```python
from build123d import *

# Parameters (mm, degrees)
ESQUISSE2_W        = 10
ESQUISSE2_H        = 8
BOSS_EXTRU_1_START = -10
BOSS_EXTRU_1_DEPTH = 10


with BuildPart() as part:
    # Esquisse2 → Révolution1 (revolve)
    with BuildSketch(Plane(origin=(0, 0, 0), x_dir=(0, 0, -1), z_dir=(1, 0, 0)), mode=Mode.PRIVATE) as r_volution1_sk:
        with Locations((5, 7)):
            Rectangle(ESQUISSE2_W, ESQUISSE2_H)
    revolve(r_volution1_sk.sketch.rotate(Axis((0, 0, 0), (0, 0, -1)), 90), axis=Axis((0, 0, 0), (0, 0, -1)))

    # Esquisse3 → Boss.-Extru.1 (add)
    with BuildSketch(Plane.XY.offset(BOSS_EXTRU_1_START)):
        with BuildLine():
            Line((0, 14), (-1.5, 10.897247359))
            ThreePointArc((-1.5, 10.897247359), (-0.751757625, 10.974281775), (0, 11))
            ThreePointArc((0, 11), (0.751757625, 10.974281775), (1.5, 10.897247359))
            Line((1.5, 10.897247359), (0, 14))
        make_face()
        with BuildLine():
            Line((3.944255796, 13.432901631), (4.509348821, 10.033233437))
            ThreePointArc((4.509348821, 10.033233437), (3.813118623, 10.317951656), (3.099058125, 10.55442271))
            ThreePointArc((3.099058125, 10.55442271), (2.370506305, 10.741540851), (1.630869901, 10.878431108))
            Line((1.630869901, 10.878431108), (3.944255796, 13.432901631))
        make_face()
        with BuildLine():
            Line((7.568971444, 11.77754946), (7.153377019, 8.356386613))
            ThreePointArc((7.153377019, 8.356386613), (6.565563427, 8.825722457), (5.947048992, 9.253788861))
            ThreePointArc((5.947048992, 9.253788861), (5.300725912, 9.63858417), (4.629616421, 9.978309065))
            Line((4.629616421, 9.978309065), (7.568971444, 11.77754946))
        make_face()
        with BuildLine():
            Line((10.580494041, 9.168050275), (9.217881154, 6.002555042))
            ThreePointArc((9.217881154, 6.002555042), (8.78610533, 6.618485713), (8.313245318, 7.203468073))
            ThreePointArc((8.313245318, 7.203468073), (7.80151223, 7.754766722), (7.253298952, 8.269803765))
            Line((7.253298952, 8.269803765), (10.580494041, 9.168050275))
        make_face()
        with BuildLine():
            Line((12.734847935, 5.815810182), (10.535607378, 3.16243216))
            ThreePointArc((10.535607378, 3.16243216), (10.294849232, 3.875058618), (10.005951949, 4.569565143))
            ThreePointArc((10.005951949, 4.569565143), (9.670266425, 5.242704194), (9.289362339, 5.891328146))
            Line((9.289362339, 5.891328146), (12.734847935, 5.815810182))
        make_face()
        with BuildLine():
            Line((13.857500186, 1.992407736), (10.999801351, 0.066107833))
            ThreePointArc((10.999801351, 0.066107833), (10.969565675, 0.81769732), (10.888035861, 1.565463221))
            ThreePointArc((10.888035861, 1.565463221), (10.755593145, 2.305908952), (10.572856836, 3.035572158))
            Line((10.572856836, 3.035572158), (13.857500186, 1.992407736))
        make_face()
        with BuildLine():
            Line((13.857500186, -1.992407736), (10.572856836, -3.035572158))
            ThreePointArc((10.572856836, -3.035572158), (10.755593145, -2.305908952), (10.888035861, -1.565463221))
            ThreePointArc((10.888035861, -1.565463221), (10.969565675, -0.81769732), (10.999801351, -0.066107833))
            Line((10.999801351, -0.066107833), (13.857500186, -1.992407736))
        make_face()
        with BuildLine():
            Line((12.734847935, -5.815810182), (9.289362339, -5.891328146))
            ThreePointArc((9.289362339, -5.891328146), (9.670266425, -5.242704194), (10.005951949, -4.569565143))
            ThreePointArc((10.005951949, -4.569565143), (10.294849232, -3.875058618), (10.535607378, -3.16243216))
            Line((10.535607378, -3.16243216), (12.734847935, -5.815810182))
        make_face()
        with BuildLine():
            Line((10.580494041, -9.168050275), (7.253298952, -8.269803765))
            ThreePointArc((7.253298952, -8.269803765), (7.80151223, -7.754766722), (8.313245318, -7.203468073))
            ThreePointArc((8.313245318, -7.203468073), (8.78610533, -6.618485713), (9.217881154, -6.002555042))
            Line((9.217881154, -6.002555042), (10.580494041, -9.168050275))
        make_face()
        with BuildLine():
            Line((7.568971444, -11.77754946), (4.629616421, -9.978309065))
            ThreePointArc((4.629616421, -9.978309065), (5.300725912, -9.63858417), (5.947048992, -9.253788861))
            ThreePointArc((5.947048992, -9.253788861), (6.565563427, -8.825722457), (7.153377019, -8.356386613))
            Line((7.153377019, -8.356386613), (7.568971444, -11.77754946))
        make_face()
        with BuildLine():
            Line((3.944255796, -13.432901631), (1.630869901, -10.878431108))
            ThreePointArc((1.630869901, -10.878431108), (2.370506305, -10.741540851), (3.099058125, -10.55442271))
            ThreePointArc((3.099058125, -10.55442271), (3.813118623, -10.317951656), (4.509348821, -10.033233437))
            Line((4.509348821, -10.033233437), (3.944255796, -13.432901631))
        make_face()
        with BuildLine():
            Line((0, -14), (-1.5, -10.897247359))
            ThreePointArc((-1.5, -10.897247359), (-0.751757625, -10.974281775), (0, -11))
            ThreePointArc((0, -11), (0.751757625, -10.974281775), (1.5, -10.897247359))
            Line((1.5, -10.897247359), (0, -14))
        make_face()
        with BuildLine():
            Line((-3.944255796, -13.432901631), (-4.509348821, -10.033233437))
            ThreePointArc((-4.509348821, -10.033233437), (-3.813118623, -10.317951656), (-3.099058125, -10.55442271))
            ThreePointArc((-3.099058125, -10.55442271), (-2.370506305, -10.741540851), (-1.630869901, -10.878431108))
            Line((-1.630869901, -10.878431108), (-3.944255796, -13.432901631))
        make_face()
        with BuildLine():
            Line((-7.568971444, -11.77754946), (-7.153377019, -8.356386613))
            ThreePointArc((-7.153377019, -8.356386613), (-6.565563427, -8.825722457), (-5.947048992, -9.253788861))
            ThreePointArc((-5.947048992, -9.253788861), (-5.300725912, -9.63858417), (-4.629616421, -9.978309065))
            Line((-4.629616421, -9.978309065), (-7.568971444, -11.77754946))
        make_face()
        with BuildLine():
            Line((-10.580494041, -9.168050275), (-9.217881154, -6.002555042))
            ThreePointArc((-9.217881154, -6.002555042), (-8.78610533, -6.618485713), (-8.313245318, -7.203468073))
            ThreePointArc((-8.313245318, -7.203468073), (-7.80151223, -7.754766722), (-7.253298952, -8.269803765))
            Line((-7.253298952, -8.269803765), (-10.580494041, -9.168050275))
        make_face()
        with BuildLine():
            Line((-12.734847935, -5.815810182), (-10.535607378, -3.16243216))
            ThreePointArc((-10.535607378, -3.16243216), (-10.294849232, -3.875058618), (-10.005951949, -4.569565143))
            ThreePointArc((-10.005951949, -4.569565143), (-9.670266425, -5.242704194), (-9.289362339, -5.891328146))
            Line((-9.289362339, -5.891328146), (-12.734847935, -5.815810182))
        make_face()
        with BuildLine():
            Line((-13.857500186, -1.992407736), (-10.999801351, -0.066107833))
            ThreePointArc((-10.999801351, -0.066107833), (-10.969565675, -0.81769732), (-10.888035861, -1.565463221))
            ThreePointArc((-10.888035861, -1.565463221), (-10.755593145, -2.305908952), (-10.572856836, -3.035572158))
            Line((-10.572856836, -3.035572158), (-13.857500186, -1.992407736))
        make_face()
        with BuildLine():
            Line((-13.857500186, 1.992407736), (-10.572856836, 3.035572158))
            ThreePointArc((-10.572856836, 3.035572158), (-10.755593145, 2.305908952), (-10.888035861, 1.565463221))
            ThreePointArc((-10.888035861, 1.565463221), (-10.969565675, 0.81769732), (-10.999801351, 0.066107833))
            Line((-10.999801351, 0.066107833), (-13.857500186, 1.992407736))
        make_face()
        with BuildLine():
            Line((-12.734847935, 5.815810182), (-9.289362339, 5.891328146))
            ThreePointArc((-9.289362339, 5.891328146), (-9.670266425, 5.242704194), (-10.005951949, 4.569565143))
            ThreePointArc((-10.005951949, 4.569565143), (-10.294849232, 3.875058618), (-10.535607378, 3.16243216))
            Line((-10.535607378, 3.16243216), (-12.734847935, 5.815810182))
        make_face()
        with BuildLine():
            Line((-10.580494041, 9.168050275), (-7.253298952, 8.269803765))
            ThreePointArc((-7.253298952, 8.269803765), (-7.80151223, 7.754766722), (-8.313245318, 7.203468073))
            ThreePointArc((-8.313245318, 7.203468073), (-8.78610533, 6.618485713), (-9.217881154, 6.002555042))
            Line((-9.217881154, 6.002555042), (-10.580494041, 9.168050275))
        make_face()
        with BuildLine():
            Line((-7.568971444, 11.77754946), (-4.629616421, 9.978309065))
            ThreePointArc((-4.629616421, 9.978309065), (-5.300725912, 9.63858417), (-5.947048992, 9.253788861))
            ThreePointArc((-5.947048992, 9.253788861), (-6.565563427, 8.825722457), (-7.153377019, 8.356386613))
            Line((-7.153377019, 8.356386613), (-7.568971444, 11.77754946))
        make_face()
        with BuildLine():
            Line((-3.944255796, 13.432901631), (-1.630869901, 10.878431108))
            ThreePointArc((-1.630869901, 10.878431108), (-2.370506305, 10.741540851), (-3.099058125, 10.55442271))
            ThreePointArc((-3.099058125, 10.55442271), (-3.813118623, 10.317951656), (-4.509348821, 10.033233437))
            Line((-4.509348821, 10.033233437), (-3.944255796, 13.432901631))
        make_face()
    extrude(amount=BOSS_EXTRU_1_DEPTH)


solid = part.part
```
Build history of the part. All positions in model axes, mm. A direction names the side the tool comes from. Give positions to 0.01 mm unless a question says otherwise; leave off trailing zeros. Order: outer loops, then holes, each group sorted by start corner. A loop starts at its lowest first (then second) coordinate and runs counter-clockwise, first axis right, second up. Notation, with made-up numbers: M 8,-39 L 49,-39 A16 cw 49,-18 Z; hole C 50.5,82 d7. An arc over 180 degrees is marked long. Write item = value, one per line. Start each with the question number.
(1) Slice it at A-A on x = 10. Write the cut outline in (y, z), plus the area to 3 significant figures.
(2) Slice it at C-C on x = 5.5. Write the cut outline in (y, z), plus the area to 3 significant figures.
(3) Slice it at B-B on y = -4.5. Write the cut outline in (x, z).
(4) Which spindle directions (+Z, -Z, +X, -X, +Y, -Y) get a long thin tool onto all of the face, cutting with end or side? Do faces 4 (the flat face through (-2.8, 12.17, -5.07)), 5 (the flat face through (9.91, 7.61, -5.07)), 6 (the flat face through (-2.771, -12.138, -5.07)), 7 (the flat face through (-9.89, 7.56, -5.07)). Say none if no direction does.
(5) Two-plate mould, pull along Y, no slides. Class faces 1 (the flat face through (-6.12, 10.89, -5.07)), 2 (the flat face through (-12.238, 2.507, -5.07)), 3 (the flat face through (6.12, -10.89, -5.07)): released by +Y, released by -Y, zero draft, split by the parting line, or undercut.
(6) Probe L1, parallel to X at y = 12, z = -9; L2, parallel to Y at x = -12.5, z = -0.5; L3, parallel to X at y = 10.75, z = -6. List the from-to ranges inside material, lowest first. Write a range as [from, to].
(7) Pin check, flat tips, straight feed: pin 1 Ø5 at (y, z) = (9, -9) entering from -X; pin 2 Ø6 at (y, z) = (4, -8) entering from -X; pin 3 Ø5 at (y, z) = (-10, -3.5) entering from +X; pin 4 Ø2 at (x, z) = (4, -6) entering from +Y. Stop position of each tip, or through.
Responses:
q1.outline = M -9.01,-10 L -7.82,-10 L -7.82,0 L -9.01,0 Z; M -5.88,-10 L 5.88,-10 L 5.88,0 L -5.88,0 Z; M 7.82,-10 L 9.01,-10 L 9.01,0 L 7.82,0 Z
q1.area = 141 mm2
q2.outline = M -10.51,-10 L 10.51,-10 L 10.51,0 L -10.51,0 Z
q2.area = 210 mm2
q3.outline = M -11.64,-10 L 11.64,-10 L 11.64,0 L -11.64,0 Z
q4.face_4 = +Z, -Z, +Y
q4.face_5 = +Z, -Z, +X
q4.face_6 = +Z, -Z, -Y
q4.face_7 = +Z, -Z, -X
q5.face_1 = released by +Y
q5.face_2 = undercut
q5.face_3 = released by -Y
q6.L1 = [-4.18, -2.65], [-0.97, 0.97], [2.65, 4.18]
q6.L2 = [-5.82, -5.53], [-2.42, -1.08], [1.08, 2.42], [5.53, 5.82]
q6.L3 = [-7.44, -5.89], [-4.39, 4.39], [5.89, 7.44]
q7.pin_1 = -10.58
q7.pin_2 = -13.86
q7.pin_3 = 10.58
q7.pin_4 = 13.43
